Geometry: final body of the model. Coordinates: model frame, mm. A direction names the side the tool comes from. Coordinates: 2 decimals unless noted, no trailing zeros. Write each loop counter-clockwise with the first axis right and the second up, starting at its lowest first coordinate (ties: lowest second). Pieces come first, ordered by that corner, then holes. Notation, with made-up numbers: (-5.75, -35.75) - (13.25, -35.75) arc R35 cw to (13.25, -0.75) - close; hole circle Ø1 at (64, -22.75). An arc over 180 degrees is marked (long way). Put each result on its own line as item: value.
```python
from build123d import *

# Parameters (mm, degrees)
SKETCH_3_R      = 2
EXTRUDE_1_DEPTH = 2


with BuildPart() as part:
    # 草图3 → 凸台-拉伸1 (new body)
    with BuildSketch(Plane.XY):
        with BuildLine():
            Line((-24.370679003, 23.782446214), (-30.099281566, 16.91223147))
            ThreePointArc((-30.099281566, 16.91223147), (-41.650836745, 31.233470531), (-46.819267976, 48.891999177))
            Line((-46.819267976, 48.891999177), (-52, 53.009783315))
            Line((-52, 53.009783315), (-47, 53.009783315))
            Line((-47, 53.009783315), (-45.565810046, 57.304305059))
            Line((-45.565810046, 57.304305059), (-37.81169544, 57.304305059))
            ThreePointArc((-37.81169544, 57.304305059), (-35.321249666, 38.8472782), (-24.370679003, 23.782446214))
        make_face()
        with Locations((-30.0520382, 22.957745114)):
            Circle(SKETCH_3_R, mode=Mode.SUBTRACT)
        with Locations((-42.5, 53.009783315)):
            Circle(SKETCH_3_R, mode=Mode.SUBTRACT)
    extrude(amount=EXTRUDE_1_DEPTH)


solid = part.part
```
1. Mould query, pull axis X, two halves, no side actions, for faces 3 (the cylindrical face through (-41.577, 51.235, 0.986)), 4 (the flat face through (-42, 57.304, 1)), 5 (the flat face through (-27.19, 20.4, 0.99)), 6 (the flat face through (-46.3, 55.1, 1)). Classes: +X half, -X half, draft (parallel to the pull), parting line (faces both ways), or undercut.
Answer below:
face 3: undercut
face 4: draft
face 5: +X half
face 6: -X half
2. Section query B-B (y = 54.5). Return loops of the section in (x, z).
Answer below:
outline: (-46.5, 0) - (-43.83, 0) - (-43.83, 2) - (-46.5, 2) - close; (-41.17, 0) - (-38.03, 0) - (-38.03, 2) - (-41.17, 2) - close
3. Section query D-D (y = 37). Return loops of the section in (x, z), then the cut area to 3 significant figures.
Answer below:
outline: (-44.19, 0) - (-34.52, 0) - (-34.52, 2) - (-44.19, 2) - close
area: 19.3 mm²
4. Ray query, probe 1 along Y at (x, z) = (-42.5, 1.1); probe 2 along Y at (x, z) = (-41.25, 1.55); probe 3 along Y at (x, z) = (-27, 1.8). Return the intervals inside material, ascending. Write a range as from..to.
Answer below:
probe 1: y = 32.94..51.01, 55.01..57.3
probe 2: y = 30.48..51.45, 54.57..57.3
probe 3: y = 20.63..26.19
5. Section query A-A (x = -29). Return loops of the section in (y, z), then the cut area to 3 significant figures.
Answer below:
outline: (18.23, 0) - (21.26, 0) - (21.26, 2) - (18.23, 2) - close; (24.66, 0) - (28.37, 0) - (28.37, 2) - (24.66, 2) - close
area: 13.5 mm²
6. Set-up query: faces 1 (the cylindrical face through (-41.53, 31, 0.99)), 2 (the flat face through (-50, 53.01, 1)). Return all of +Z, -Z, +X, -X, +Y, -Y with unobstructed straight access to the full face (end or side cutting, diameter ignored); none if empty.
Answer below:
face 1: +Z, -Z, -X, -Y
face 2: +Z, -Z, -X, +Y
7. Pin query (flat end, axial travel): pin 1 Ø6.5 at (x, y) = (-30.05, 22.96) entering from +Z. Return the tip coordinate at first contact, or that it passes through.
Answer below:
pin 1: stops at z = 2
8. Section query C-C (z = 0.7). Return loops of the section in (x, y), then the cut area to 3 significant figures.
Answer below:
outline: (-52, 53.01) - (-46.82, 48.89) arc R47 ccw to (-30.1, 16.91) - (-24.37, 23.78) arc R38.05 cw to (-37.81, 57.3) - (-45.57, 57.3) - (-47, 53.01) - close; hole circle Ø4 at (-42.5, 53.01); hole circle Ø4 at (-30.05, 22.96)
area: 354 mm²
